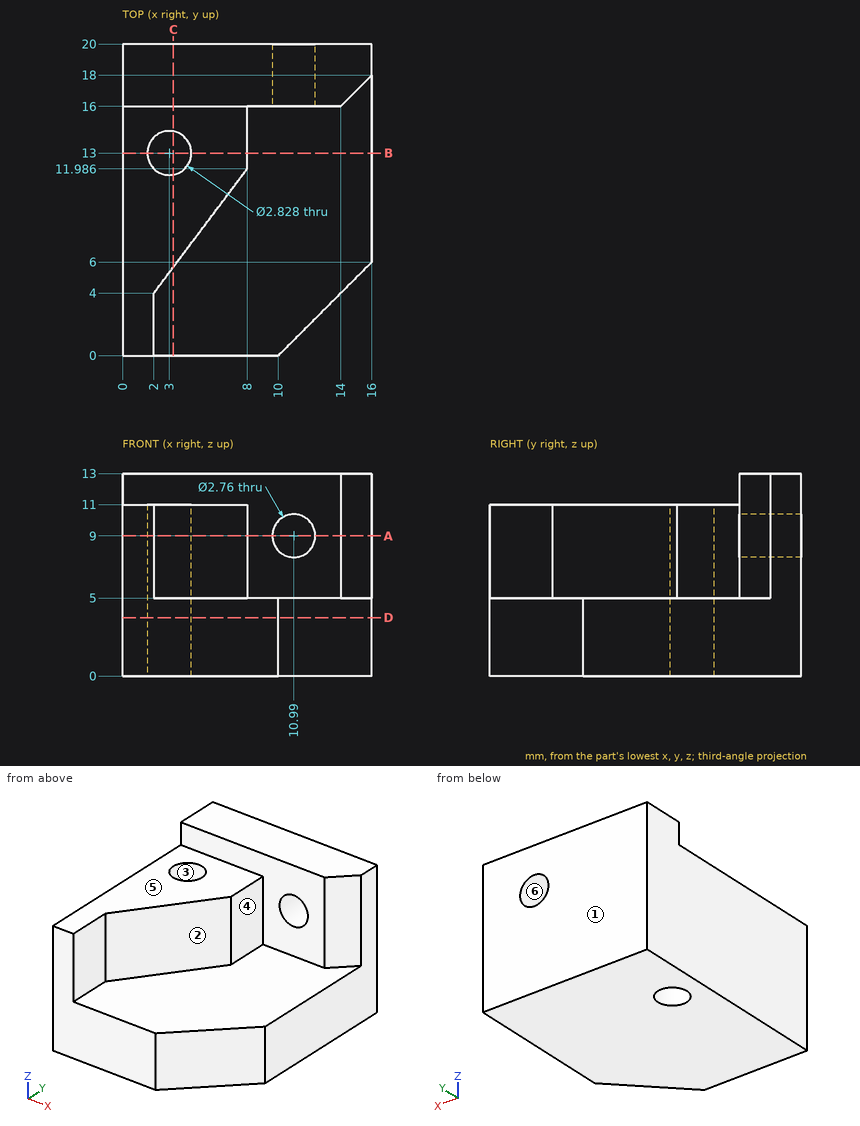
Could you check a few things on this drawing? It's one solid part, dimensions in mm from its lowest x, y, z. A direction names the side the tool comes from. Round coordinates to 2 decimals unless told otherwise and drop trailing zeros. Loops run counter-clockwise (first coordinate to the right, second up) from the corner with the lowest first, then second, coordinate; pieces in that order, holes last. Notation, with made-up numbers: (80.25, 9) -> (129.25, 9) arc R7 cw to (129.25, 19) -> close; hole circle Ø10 at (79, -22). An arc over 180 degrees is marked (long way). One line per item, written item: value. Start each with the question number.
1. If I drill on probe 1 along X at (y, z) = (13, 3) (1 decimal); probe 2 along X at (y, z) = (13, 6.5) (1 decimal); probe 3 along Y at (x, z) = (3, 2) (1 decimal), over which ranges is the centre line in solid material (lowest first)?
2. If we section it at D-D, the plane z = 3.75: Write out the boundary of the cut face in (x, y) (1 decimal).
3. If we section it at A-A, the plane z = 9: Write out the boundary of the cut face in (x, y) (1 decimal), then the cut area to 3 significant figures.
4. If we section it at C-C, the plane x = 3.25: Write out the boundary of the cut face in (y, z), then the cut area to 3 significant figures.
5. If we section it at B-B, the plane y = 13: Write out the boundary of the cut face in (x, z) (1 decimal).
6. If we mould it in two halves opening along X, with no side actions, what happens to the marked faces 3, 4, 5 and 6? For each: pulls with the +X half, pulls with the -X half, needs draft (parallel to the pull), parting line crosses it, or undercut.
7. For the marked faces 1 and 2, which set-ups out of +Z, -Z, +X, -X, +Y, -Y let a thin tool reach every point of the face, with its end or its side?
8. For pin 1 (5 mm diameter, centred on y = 13, z = 11.5, fed in from +X); pin 2 (6.5 mm diameter, centred on x = 3.5, y = 6, fed in from +Z); pin 3 (1.2 mm diameter, centred on y = 2.5, z = 9, fed in from +X), each with a flat end and sliding along its axis, tell me the tip position at first contact or that it passes through.
Calculated:
1. probe 1: x = 0 to 1.6, 4.4 to 16
1. probe 2: x = 0 to 1.6, 4.4 to 8
1. probe 3: y = 0 to 11.6, 14.4 to 20
2. outline: (0, 0) -> (10, 0) -> (16, 6) -> (16, 20) -> (0, 20) -> close; hole circle Ø2.8 at (3, 13)
3. outline: (0, 0) -> (2, 0) -> (2, 4) -> (8, 12) -> (8, 16) -> (9.6, 16) -> (9.6, 20) -> (0, 20) -> close; (12.4, 16) -> (14, 16) -> (16, 18) -> (16, 20) -> (12.4, 20) -> close; hole circle Ø2.8 at (3, 13)
3. area: 125 mm²
4. outline: (0, 0) -> (11.61, 0) -> (11.61, 11) -> (5.66, 11) -> (5.66, 5) -> (0, 5) -> close; (14.39, 0) -> (20, 0) -> (20, 13) -> (16, 13) -> (16, 11) -> (14.39, 11) -> close
4. area: 163 mm²
5. outline: (0, 0) -> (1.6, 0) -> (1.6, 11) -> (0, 11) -> close; (4.4, 0) -> (16, 0) -> (16, 5) -> (8, 5) -> (8, 11) -> (4.4, 11) -> close
6. face 3: undercut
6. face 4: pulls with the +X half
6. face 5: needs draft
6. face 6: undercut
7. face 1: +Z, -Z, +X, -X, +Y
7. face 2: +Z, +X, -Y
8. pin 1: stops at x = 8
8. pin 2: stops at z = 11
8. pin 3: stops at x = 2
